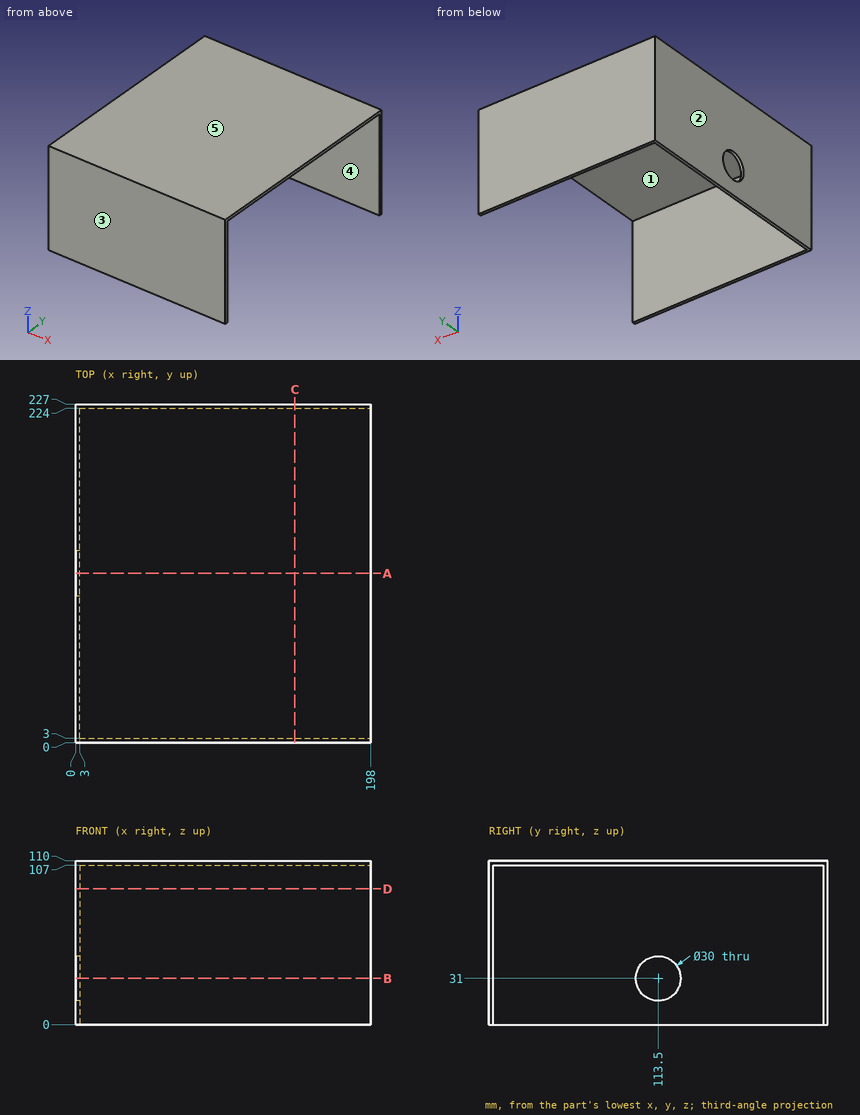
Source: three-view drawing plus pictorial views. Frame: mm from the lowest corner of the part. A direction names the side the tool comes from. Coordinates: 2 decimals unless noted, no trailing zeros. Loops run counter-clockwise (first coordinate to the right, second up) from the corner with the lowest first, then second, coordinate; pieces in that order, holes last. Notation, with made-up numbers: (5, -12) - (13, -12) arc R12 ccw to (13, -8) - close; hole circle Ø7 at (23, 72.25). An arc over 180 degrees is marked (long way). One line per question, with ' | ' between items.
1) Section A-A, the plane y = 113.5. Return loops of the section in (x, z).
Report:
outline: (0, 0) - (3, 0) - (3, 16) - (0, 16) - close; (0, 46) - (3, 46) - (3, 107) - (198, 107) - (198, 110) - (0, 110) - close
2) Pull-direction query (Y, two-part tool) for the marked faces 3, 4 and 5; classes: released by +Y, released by -Y, zero draft, split by the parting line, or undercut.
Report:
face 3: released by -Y | face 4: undercut | face 5: zero draft
3) Section B-B, the plane z = 31. Return loops of the section in (x, y), then the cut area to 3 significant figures.
Report:
outline: (0, 0) - (198, 0) - (198, 3) - (3, 3) - (3, 98.5) - (0, 98.5) - close; (0, 128.5) - (3, 128.5) - (3, 224) - (198, 224) - (198, 227) - (0, 227) - close | area: 1,760 mm²
4) Line query: line 1 along Y through (x, z) = (85.5, 47.5); line 2 along Z through (x, y) = (2, 113); line 3 along Z through (x, y) = (89, 75.5). Output: solid intervals per line, ascending.
Report:
line 1: y = 0 to 3, 224 to 227 | line 2: z = 0 to 16.01, 45.99 to 110 | line 3: z = 107 to 110
5) Section C-C, the plane x = 147. Return loops of the section in (y, z), then the cut area to 3 significant figures.
Report:
outline: (0, 0) - (3, 0) - (3, 107) - (224, 107) - (224, 0) - (227, 0) - (227, 110) - (0, 110) - close | area: 1,320 mm²
6) Section D-D, the plane z = 91. Return loops of the section in (x, y).
Report:
outline: (0, 0) - (198, 0) - (198, 3) - (3, 3) - (3, 224) - (198, 224) - (198, 227) - (0, 227) - close
7) First-contact query: P1, Ø6, axis at x = 139, y = 27.5, coming from the -Z side; P2, Ø3, axis at y = 91, z = 98, coming from the +X side. Flat tips, straight axial feed; report the tip coordinate or a pass-through.
Report:
P1: stops at z = 107 | P2: stops at x = 3
8) Set-up query: the marked faces 1 and 2. Return all of +Z, -Z, +X, -X, +Y, -Y with unobstructed straight access to the full face (end or side cutting, diameter ignored); none if empty.
Report:
face 1: -Z, +X | face 2: +Z, -Z, -X, +Y, -Y
